Check sheet for the modelled part. Datum: model origin and axes. Units: mm. A direction names the side the tool comes from. Give positions to 0.01 mm unless a question says otherwise; leave off trailing zeros. Order: outer loops, then holes, each group sorted by start corner. A loop starts at its lowest first (then second) coordinate and runs counter-clockwise, first axis right, second up. Notation, with made-up numbers: (-7, -5) -> (16, -5) arc R15 ccw to (16, 8) -> close; hole circle Ø6 at (28, 45). An arc over 180 degrees is marked (long way). Write each question's results on one line, items separated by ' | '.
from build123d import *

# Parameters (mm, degrees)
F0_R     = 11.5
F1_DEPTH = 10
F2_R     = 5
F3_R     = 5.25
F4_DEPTH = 10.001


with BuildPart() as f1:
    # F0 (on Front) → F1 (new body)
    with BuildSketch(Plane.XZ):
        Polygon((75, -100), (75, 100), (0, 100), (-75, 100), (-75, -100), (-20, -100), (-20, -40), (20, -40), (20, -100), align=None)
        with Locations((-37.5, 65)):
            Circle(F0_R, mode=Mode.SUBTRACT)
        with Locations((37.5, 65)):
            Circle(F0_R, mode=Mode.SUBTRACT)
        Polygon((0, 100), (75, 100), (0, 175), align=None)
        Polygon((-75, 100), (0, 100), (0, 175), align=None)
    extrude(amount=F1_DEPTH)

    # F2
    f2_edges = [f1.edges().sort_by_distance(p)[0] for p in [
        (-20, -5, -40),
        (20, -5, -40),
    ]]
    fillet(f2_edges, radius=F2_R)

    # F3 (on face) → F4 (cut, through all)
    with BuildSketch(Plane(origin=(0, 0, 0), x_dir=(-1, 0, 0), z_dir=(0, 1, 0))):
        with Locations((0, 15)):
            Circle(F3_R)
    extrude(amount=-F4_DEPTH, mode=Mode.SUBTRACT)


solid = f1.part
1. Access from +Z, -Z, +X, -X, +Y, -Y to the whole of each face (thin tool, end or side, straight path). Record for faces 1 (the cylindrical face through (18, -5, -41)), 2 (the flat face through (-1, -10, 39)).
Verdict:
face 1: -Z, +Y, -Y | face 2: +Z, -Z, +X, -X, -Y
2. Section check B-B on z = 65. Record the cut outline in (x, y).
Verdict:
outline: (-75, -10) -> (-49, -10) -> (-49, 0) -> (-75, 0) -> close; (-26, -10) -> (26, -10) -> (26, 0) -> (-26, 0) -> close; (49, -10) -> (75, -10) -> (75, 0) -> (49, 0) -> close
3. Section check C-C on y = -5.75. Record the cut outline in (x, z).
Verdict:
outline: (-75, -100) -> (-20, -100) -> (-20, -45) arc R5 cw to (-15, -40) -> (15, -40) arc R5 cw to (20, -45) -> (20, -100) -> (75, -100) -> (75, 100) -> (0, 175) -> (-75, 100) -> close; hole circle Ø23 at (-37.5, 65); hole circle Ø10.5 at (0, 15); hole circle Ø23 at (37.5, 65)
4. Gauge pin test, flat ends, axial feed: pin 1 Ø2 at (x, y) = (-6.5, -4.5) entering from -Z; pin 2 Ø14 at (x, z) = (-37.5, 65) entering from +Y; pin 3 Ø1 at (x, y) = (4, -8) entering from +Z. Record the tip position at first contact, or that the pin passes through.
Verdict:
pin 1: stops at z = -40 | pin 2: passes through | pin 3: stops at z = 171.5
5. Mould release check, pull along X, two halves, no side actions. Record for faces 3 (the cylindrical face through (-39.993, -4.93, 53.773)), 4 (the flat face through (-48, -5, -100)), 5 (the flat face through (75, -5, -1)): +X half, -X half, draft (parallel to the pull), parting line (faces both ways), or undercut.
Verdict:
face 3: undercut | face 4: draft | face 5: +X half
6. Section check D-D on x = -37.5. Record the cut outline in (y, z).
Verdict:
outline: (-10, -100) -> (0, -100) -> (0, 53.5) -> (-10, 53.5) -> close; (-10, 76.5) -> (0, 76.5) -> (0, 137.5) -> (-10, 137.5) -> close
7. Material ranges on probe 1 along X at (y, z) = (-1.5, 59.5); probe 2 along Z at (x, y) = (-37.5, -3.25); probe 3 along Z at (x, y) = (-43, -2.5), recorded low to high. Write a range as from..to.
Verdict:
probe 1: x = -75..-47.6, -27.4..27.4, 47.6..75 | probe 2: z = -100..53.5, 76.5..137.5 | probe 3: z = -100..54.9, 75.1..132
8. Section check A-A on z = -59. Record the cut outline in (x, y).
Verdict:
outline: (-75, -10) -> (-20, -10) -> (-20, 0) -> (-75, 0) -> close; (20, -10) -> (75, -10) -> (75, 0) -> (20, 0) -> close
